```python
from build123d import *

# Parameters (mm, degrees)
F1_DEPTH = 48.26
F2_DEPTH = 28.448
F3_DEPTH = 17.272
F4_W     = 25.4
F4_H     = 10.16
F5_DEPTH = 25.4
F6_R     = 6.35
F7_DEPTH = 48.261


with BuildPart() as f1:
    # F0 (on Top) → F1 (new body)
    with BuildSketch(Plane.XY):
        Polygon((-12.7, 0), (0, 0), (35.56, 0), (48.26, 0), (48.26, 29.835004), (35.56, 29.835004), (35.56, 19.675004), (0, 19.675004), (0, 29.835004), (-12.7, 29.835004), align=None)
    extrude(amount=F1_DEPTH)

    # F0 (on Top) → F2 (join)
    with BuildSketch(Plane.XY):
        Polygon((35.56, 0), (0, 0), (0, -60.136137), (6.63483, -71.628), (28.92517, -71.628), (35.56, -60.136137), align=None)
    extrude(amount=F2_DEPTH)

    # F0 (on Top) → F3 (join)
    with BuildSketch(Plane.XY):
        Polygon((28.92517, -71.628), (6.63483, -71.628), (17.78, -90.932), align=None)
    extrude(amount=F3_DEPTH)

    # F4 (on face) → F5 (cut)
    with BuildSketch(Plane.XZ):
        with Locations((17.78, 43.18)):
            Rectangle(F4_W, F4_H)
    extrude(amount=-F5_DEPTH, mode=Mode.SUBTRACT)

    # F6 (on face) → F7 (cut, through all)
    with BuildSketch(Plane(origin=(0, 0, 0), x_dir=(0, -1, 0), z_dir=(-1, 0, 0))):
        with Locations((35.052, 14.224)):
            Circle(F6_R)
    extrude(amount=-F7_DEPTH, mode=Mode.SUBTRACT)


solid = f1.part
```
Work out the finished part from the listing and answer in its coordinate system (mm). A direction names the side the tool comes from. Round coordinates to 2 decimals unless told otherwise and drop trailing zeros. Write each loop counter-clockwise with the first axis right and the second up, starting at its lowest first coordinate (ties: lowest second). Pieces come first, ordered by that corner, then holes.
1) A cutting plane is placed at B-B on x = 21. Determine the outline of the cut face in (y, z) (3 decimals), and give its area (3 significant figures).
2) A cutting plane is placed at D-D on z = 11.5. Determine the outline of the cut face in (x, y) (3 decimals).
3) Consider probe 1 along Y at (x, z) = (-3.5, 8.5) (3 decimals); probe 2 along X at (y, z) = (-49, 21.5); probe 3 along Z at (x, y) = (16, -17.5). Determine where each line is inside the solid, lowest interval first.
4) Flat-ended cylindrical pins translate along their axes: P1, Ø1.5, axis at x = 17, y = 12.5, coming from the +Z side; P2, Ø8, axis at x = 1.5, y = -58.5, coming from the -Z side; P3, Ø8, axis at x = 22, y = -50.5, coming from the +Z side; P4, Ø2, axis at x = 34.5, z = 11, coming from the +Y side (3 decimals). Find the tip coordinate at first contact, or state that the pin passes through.
5) A cutting plane is placed at C-C on y = -39.5. Determine the outline of the cut face in (x, z).
6) Which of the six approach directions +Z, -Z, +X, -X, +Y, -Y give full straight-line access (tool end or side, diameter ignored) to faces 4 (the face through (35.56, 25, 24)), 5 (the face through (18, -79, 17.272)), 6 (the face through (30.48, 10, 43))?
7) A cutting plane is placed at A-A on z = 32. Determine the outline of the cut face in (x, y) (3 decimals), and give its area (3 significant figures).
8) Determine the mould class of faces 1 (the face through (18, -71.628, 23)), 2 (the face through (18, -35, 28.448)), 3 (the face through (17.53, -41.11, 16.13)) for opening direction Y: pulls with the +Y half, pulls with the -Y half, needs draft (parallel to the pull), parting line crosses it, or undercut.
Entries:
1. outline: (-85.355, 0) - (19.675, 0) - (19.675, 38.1) - (0, 38.1) - (0, 28.448) - (-71.628, 28.448) - (-71.628, 17.272) - (-85.355, 17.272) - close; hole circle Ø12.7 at (-35.052, 14.224)
1. area: 2,900 mm2
2. outline: (-12.7, 0) - (0, 0) - (0, -29.316) - (35.56, -29.316) - (35.56, 0) - (48.26, 0) - (48.26, 29.835) - (35.56, 29.835) - (35.56, 19.675) - (0, 19.675) - (0, 29.835) - (-12.7, 29.835) - close; (0, -60.136) - (17.78, -90.932) - (35.56, -60.136) - (35.56, -40.788) - (0, -40.788) - close
3. probe 1: y = 0 to 29.835
3. probe 2: x = 0 to 35.56
3. probe 3: z = 0 to 28.45
4. P1: stops at z = 38.1
4. P2: stops at z = 0
4. P3: stops at z = 28.45
4. P4: stops at y = 19.675
5. outline: (0, 0) - (35.56, 0) - (35.56, 9.69) - (0, 9.69) - close; (0, 18.76) - (35.56, 18.76) - (35.56, 28.45) - (0, 28.45) - close
6. face 4: +Z, -Z, +Y
6. face 5: +Z, +X, -X, -Y
6. face 6: +Z, +Y, -Y
7. outline: (-12.7, 0) - (48.26, 0) - (48.26, 29.835) - (35.56, 29.835) - (35.56, 19.675) - (0, 19.675) - (0, 29.835) - (-12.7, 29.835) - close
7. area: 1,460 mm2
8. face 1: pulls with the -Y half
8. face 2: needs draft
8. face 3: undercut
